Geometry check sheet. Reference: the model listing, model coordinates, mm. A direction names the side the tool comes from. Coordinates: 2 decimals unless noted, no trailing zeros. Loops run counter-clockwise (first coordinate to the right, second up) from the corner with the lowest first, then second, coordinate; pieces in that order, holes last. Notation, with made-up numbers: M 73.5,4 L 77.5,4 A26 cw 77.5,29 Z; hole C 26,55.5 d9. An arc over 180 degrees is marked long. Use CSV: the item, a comma, the result in double quotes.
```python
from build123d import *

# Parameters (mm, degrees)
SZKIC1_R                    = 8
DODANIE_WYCI_GNI_CIE1_DEPTH = 55
SFAZOWANIE1_SIZE            = 0.5
SZKIC2_R                    = 3
WYTNIJ_WYCI_GNI_CIE1_DEPTH  = 10
WYTNIJ_WYCI_GNI_CIE1_TAPER  = 5


with BuildPart() as part:
    # Szkic1 → Dodanie-wyciągnięcie1 (new body, symmetric)
    with BuildSketch(Plane.XY):
        with Locations((-33.610628805, 0)):
            Circle(SZKIC1_R)
    extrude(amount=DODANIE_WYCI_GNI_CIE1_DEPTH, both=True)

    # Sfazowanie1
    sfazowanie1_edges = [part.edges().sort_by_distance(p)[0] for p in [
        (-41.610628805, 0, -55),
        (-41.610628805, 0, 55),
    ]]
    chamfer(sfazowanie1_edges, length=SFAZOWANIE1_SIZE)

    # Szkic2 → Wytnij-wyciągnięcie1 (cut)
    with BuildSketch(Plane.ZY.offset(41.610628805)):
        with Locations((50.349966255, 0)):
            Circle(SZKIC2_R)
    extrude(amount=-WYTNIJ_WYCI_GNI_CIE1_DEPTH, taper=WYTNIJ_WYCI_GNI_CIE1_TAPER, mode=Mode.SUBTRACT)


solid = part.part
```
1. Gauge pin test, flat ends, axial feed: P1, Ø1, axis at x = -29.5, z = 27.5, coming from the +Y side; P2, Ø1.5, axis at y = 1.5, z = 25.5, coming from the +X side; P3, Ø1, axis at x = -37.5, z = -41.5, coming from the +Y side. Record the tip position at first contact, or that the pin passes through.
The answers:
P1,"y = 7.14"
P2,"x = -25.65"
P3,"y = 7.25"
2. Release check for a two-part mould opening along Y. For faces 1 (the conical face through (-36.541, 0.768, 52.788)), 2 (the flat face through (-34, 0, 55)), 3 (the cylindrical face through (-26.22, -3.06, 0.76)) record: +Y half, -Y half, draft (parallel to the pull), parting line (faces both ways), or undercut.
The answers:
face 1,"undercut"
face 2,"draft"
face 3,"parting line"
3. Set-up check for faces 4 (the flat face through (-31.611, 0, 50)), 5 (the flat face through (-34, 0, -55)): record each of +Z, -Z, +X, -X, +Y, -Y from which the full face is reachable in a straight line by a thin tool's end or side.
The answers:
face 4,"-X"
face 5,"-Z, +X, -X, +Y, -Y"
4. Thickness scan on line 1 (Y direction, x = -41, z = 49); line 2 (Z direction, x = -32.75, y = 1.5); line 3 (Z direction, x = -26.25, y = -1.5). Record the ranges inside material, lowest first. Write a range as [from, to].
The answers:
line 1,"[-3.07, -2.62], [2.62, 3.07]"
line 2,"[-55, 48.71], [51.99, 55]"
line 3,"[-54.99, 54.99]"
5. Section check A-A, the plane z = -39.5. Record the cut outline in (x, y).
The answers:
outline,"C -33.61,0 d16"
